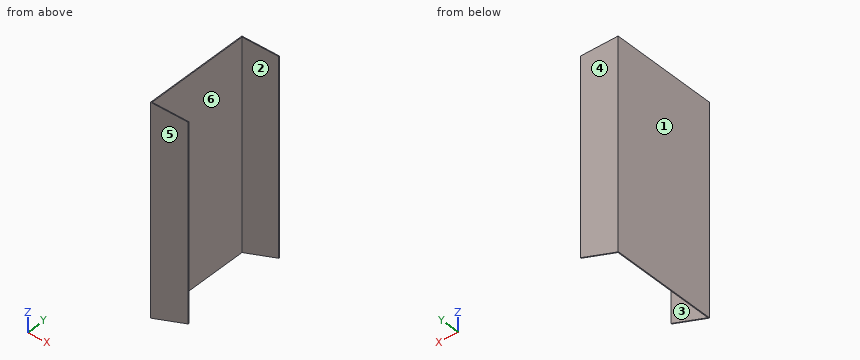
from build123d import *

# Parameters (mm, degrees)
BOSS_EXTRUDE1_DEPTH      = 21.59
BOSS_EXTRUDE1_DEPTH_BACK = 21.59
SKETCH3_W                = 241.554
SKETCH3_H                = 122.428
SHELL2_T                 = -1.016
CUT_EXTRUDE2_DEPTH       = 272.66721959
CUT_EXTRUDE2_DEPTH_BACK  = 272.66721959
MOVE_START               = -1.905
MOVE_FACE1_DEPTH         = 1.905


# Read off the part's stored shape, not the designer's step: Move Face1
with BuildPart() as part:
    # Sketch3 → Boss-Extrude1 (new, two sides: drawn at the far end of the back side and taken through both)
    with BuildSketch(Plane(origin=(0, 0, 0), x_dir=(0, 0, -1), z_dir=(1, 0, 0)).offset(-BOSS_EXTRUDE1_DEPTH_BACK)):
        with Locations((120.777, 61.214)):
            Rectangle(SKETCH3_W, SKETCH3_H)
    extrude(amount=BOSS_EXTRUDE1_DEPTH + BOSS_EXTRUDE1_DEPTH_BACK)

    # Shell2
    shell2_openings = [part.faces().sort_by_distance(p)[0] for p in [
        (21.59, 61.214, -120.777),
        (0, 61.214, -241.554),
        (0, 61.214, 0),
    ]]
    offset(amount=SHELL2_T, openings=shell2_openings, kind=Kind.INTERSECTION)

    # Sketch8 → Cut-Extrude2 (cut, two sides: drawn at the far end of the back side and taken through both)
    with BuildSketch(Plane(origin=(0, 122.428, 0), x_dir=(1, 0, 0), z_dir=(0, 1, 0)).offset(-CUT_EXTRUDE2_DEPTH_BACK)):
        Polygon((-490.808059193, 412.705200685), (-20.574, 241.554), (21.59, 226.207559042), (491.824059193, 55.056358358), (834.126460562, 995.524476744), (-148.505657824, 1353.173319071), align=None)
    extrude(amount=CUT_EXTRUDE2_DEPTH + CUT_EXTRUDE2_DEPTH_BACK, mode=Mode.SUBTRACT)

    # Move Face1 outline → Move Face1 (cut)
    with BuildSketch(Plane.XY.offset(MOVE_START)):
        Polygon((-21.59, 0), (21.59, 0), (21.59, 1.016), (-20.574, 1.016), (-20.574, 121.412), (21.59, 121.412), (21.59, 122.428), (-21.59, 122.428), align=None)
    extrude(amount=MOVE_FACE1_DEPTH, mode=Mode.SUBTRACT)


solid = part.part
Work out the finished part from the listing and answer in its coordinate system (mm). Face numbers are marked on the shaded views. A direction names the side the tool comes from. Round coordinates to 2 decimals unless told otherwise and drop trailing zeros. Write each loop counter-clockwise with the first axis right and the second up, starting at its lowest first coordinate (ties: lowest second). Pieces come first, ordered by that corner, then holes. Notation, with made-up numbers: (26, -30.75) - (58, -30.75) arc R7 cw to (58, -19.75) - close; hole circle Ø3 at (1.25, -20). An arc over 180 degrees is marked (long way). Answer in a Markdown table with one row per item. Add a question column.
1. For the marked faces 5 and 6, determine the directions among +Z, -Z, +X, -X, +Y, -Y from which every point of the face is accessible in a straight line to the end or side of a thin tool.
2. The mould has two halves that part along Y. Classify the marked faces 1, 2, 3 and 4: +Y half, -Y half, draft (parallel to the pull), parting line (faces both ways), or undercut.
3. Given pin 1 (12 mm diameter, centred on x = 0.5, z = -208, fed in from -Y); pin 2 (3 mm diameter, centred on y = 13, z = -179, fed in from +X), each flat-ended and moving along its own axis, determine where each tip first touches the part or whether it passes through.
4. Find the intervals of material crossed by line 1 along Y through (x, z) = (7.5, -49.5); line 2 along X through (y, z) = (17, -87.5), in increasing order. Write a range as from..to.
5. A cutting plane is placed at C-C, the plane x = 12. Determine the outline of the cut face in (y, z) (3 decimals).
6. A cutting plane is placed at D-D, the plane y = 88. Determine the outline of the cut face in (x, z) (3 decimals).
7. A cutting plane is placed at A-A, the plane x = -14. Determine the outline of the cut face in (y, z) (3 decimals), and give its area (3 significant figures).
8. A cutting plane is placed at B-B, the plane z = -200. Determine the outline of the cut face in (x, y), and give its area (3 significant figures).
Worked out:
| question | item | result |
|---|---|---|
| 1 | face 5 | +Z, -Z, +X, -X, -Y |
| 1 | face 6 | +Z, -Z, +X |
| 2 | face 1 | draft |
| 2 | face 2 | undercut |
| 2 | face 3 | undercut |
| 2 | face 4 | +Y half |
| 3 | pin 1 | y = 0 |
| 3 | pin 2 | x = -20.57 |
| 4 | line 1 | 0..1.02, 121.41..122.43 |
| 4 | line 2 | -21.59..-20.57 |
| 5 | outline | (0, -229.698) - (1.016, -229.698) - (1.016, -1.905) - (0, -1.905) - close; (121.412, -229.698) - (122.428, -229.698) - (122.428, -1.905) - (121.412, -1.905) - close |
| 6 | outline | (-21.59, -241.554) - (-20.574, -241.554) - (-20.574, -1.905) - (-21.59, -1.905) - close |
| 7 | outline | (0, -239.161) - (1.016, -239.161) - (1.016, -1.905) - (0, -1.905) - close; (121.412, -239.161) - (122.428, -239.161) - (122.428, -1.905) - (121.412, -1.905) - close |
| 7 | area | 482 mm^2 |
| 8 | outline | (-21.59, 0) - (21.59, 0) - (21.59, 1.02) - (-20.57, 1.02) - (-20.57, 121.41) - (21.59, 121.41) - (21.59, 122.43) - (-21.59, 122.43) - close |
| 8 | area | 210 mm^2 |
